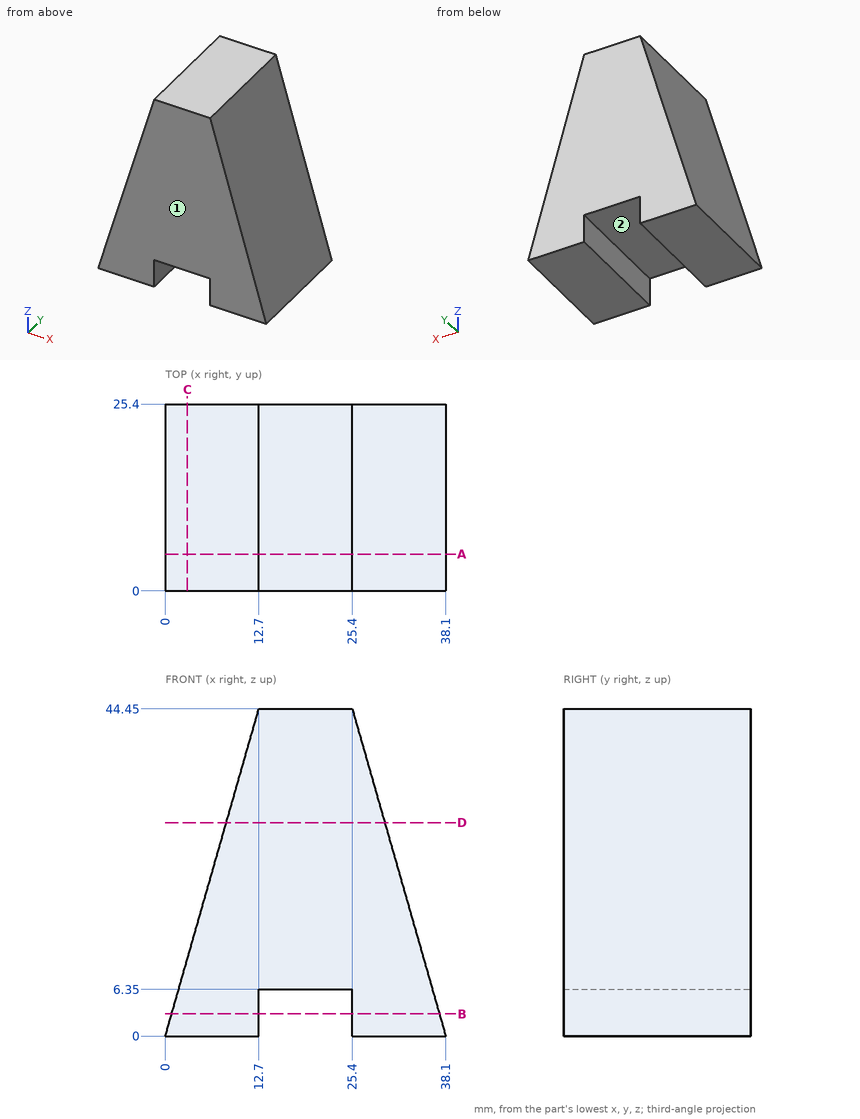
Geometry: see drawing. Coordinates: mm, zero at the bounding-box minimum. A direction names the side the tool comes from. Coordinates: 2 decimals unless noted, no trailing zeros. Write each loop counter-clockwise with the first axis right and the second up, starting at its lowest first coordinate (ties: lowest second). Pieces come first, ordered by that corner, then holes. Notation, with made-up numbers: (89, 64) - (103, 64) arc R13 ccw to (103, 77) - close; hole circle Ø9 at (86.5, 63.5). An arc over 180 degrees is marked (long way). Put each result on its own line as item: value. Start each with the question number.
1) Contact query for flat-ended pins moving along their axis: pin 1 (1.5 mm diameter, centred on y = 14, z = 5, fed in from -X); pin 2 (3 mm diameter, centred on y = 7.5, z = 4.5, fed in from +X); pin 3 (1.5 mm diameter, centred on y = 9, z = 27.5, fed in from -X). Output: stop coordinate, or through.
2) Ray query, L1, parallel to Z at x = 22, y = 4.5; L2, parallel to X at y = 21.75, z = 5; L3, parallel to X at y = 22.75, z = 2.5. Return the intervals inside material, ascending.
3) Cut plane B-B (z = 3). Return the cut outline in (x, y), plus the area to 3 significant figures.
4) Cut plane C-C (x = 3). Return the cut outline in (y, z).
5) Reachability of the marked faces 1 and 2 from +Z, -Z, +X, -X, +Y, -Y: full face, straight path, thin tool, end or side. Return the list, or none.
6) Cut plane D-D (z = 29). Return the cut outline in (x, y).
7) Cut plane A-A (y = 5). Return the cut outline in (x, z).
Resolved:
1. pin 1: stops at x = 1.21
1. pin 2: stops at x = 37.24
1. pin 3: stops at x = 7.64
2. L1: z = 6.35 to 44.45
2. L2: x = 1.43 to 12.7, 25.4 to 36.67
2. L3: x = 0.71 to 12.7, 25.4 to 37.39
3. outline: (0.86, 0) - (12.7, 0) - (12.7, 25.4) - (0.86, 25.4) - close; (25.4, 0) - (37.24, 0) - (37.24, 25.4) - (25.4, 25.4) - close
3. area: 602 mm2
4. outline: (0, 0) - (25.4, 0) - (25.4, 10.5) - (0, 10.5) - close
5. face 1: +Z, -Z, +X, -X, -Y
5. face 2: -Z, +Y, -Y
6. outline: (8.29, 0) - (29.81, 0) - (29.81, 25.4) - (8.29, 25.4) - close
7. outline: (0, 0) - (12.7, 0) - (12.7, 6.35) - (25.4, 6.35) - (25.4, 0) - (38.1, 0) - (25.4, 44.45) - (12.7, 44.45) - close
